```python
from build123d import *

# Parameters (mm, degrees)
F0_W     = 74.9250464141
F0_H     = 66.6232015938
F1_DEPTH = 25.4
F3_DEPTH = 84.074
F4_R     = 1.27


with BuildPart() as f1:
    # F0 (on Top) → F1 (new body)
    with BuildSketch(Plane.XY):
        with Locations((-4.7604274005, 6.0135135427)):
            Rectangle(F0_W, F0_H)
    extrude(amount=F1_DEPTH)

    # F2 (on face) → F3 (cut)
    with BuildSketch(Plane.YZ.offset(32.7020958066)):
        Polygon((25.5974382162, 18.2015541941), (-8.4044123068, 18.2015541941), (1.5848320909, 7.8281089664), (17.7213028073, 7.8281089664), align=None)
    extrude(amount=-F3_DEPTH, mode=Mode.SUBTRACT)

    # F4
    f4_edges = [f1.edges().sort_by_distance(p)[0] for p in [
        (-4.760427, 1.584832, 7.828109),
        (-4.760427, 25.597438, 18.201554),
    ]]
    fillet(f4_edges, radius=F4_R)


solid = f1.part
```
Part model, mm, in its own coordinate system. A direction names the side the tool comes from. Give positions to 0.01 mm unless a question says otherwise; leave off trailing zeros. Write each loop counter-clockwise with the first axis right and the second up, starting at its lowest first coordinate (ties: lowest second). Pieces come first, ordered by that corner, then holes. Notation, with made-up numbers: (77.5, -11) -> (89.5, -11) arc R30 cw to (89.5, 22) -> close; hole circle Ø9 at (73.5, -1). An arc over 180 degrees is marked (long way). Put each result on its own line as item: value. Start each with the question number.
Item 1: Cut at C-C (z = 11). List the corners of the cut face in (x, y), then the cut area to 3 significant figures.
Item 2: Which spindle directions (+Z, -Z, +X, -X, +Y, -Y) get a long thin tool onto all of the face, cutting with end or side? Do faces 1 (the face through (-4.236, -3.664, 13.279)), 2 (the face through (-5, 6, 25.4)). Say none if no direction does.
Item 3: Pin check, flat tip, straight feed: pin 1 Ø25 at (x, y) = (-18.5, 14) entering from -Z. Stop position of the tip, or through.
Item 4: Wall check: L1, parallel to Z at x = -11.5, y = 7; L2, parallel to Z at x = -12, y = 1; L3, parallel to Y at x = -12, z = 9. Give the ranges that are in metal, low to high. Write a range as [from, to].
Item 5: Cut at A-A (y = 7.5). List the corners of the cut face in (x, z).
Item 6: Cut at B-B (x = -17). List the corners of the cut face in (y, z), then the cut area to 3 significant figures.
Item 7: Pull direction Y, two halves, no side cores. Call faces 3 (the face through (-5, 39.325, 13)), 4 (the face through (-5.28, 24.17, 17.51)), 5 (the face through (-5, -27.298, 13)): pulls with the +Y half, pulls with the -Y half, needs draft (parallel to the pull), parting line crosses it, or undercut.
Answer list:
1. outline: (-42.22, -27.3) -> (32.7, -27.3) -> (32.7, -1.47) -> (-42.22, -1.47) -> close; (-42.22, 20.13) -> (32.7, 20.13) -> (32.7, 39.33) -> (-42.22, 39.33) -> close
1. area: 3,370 mm2
2. face 1: +X, -X
2. face 2: +Z, +X, -X, +Y, -Y
3. pin 1: stops at z = 0
4. L1: z = [0, 7.83], [18.2, 25.4]
4. L2: z = [0, 8.44], [18.2, 25.4]
4. L3: y = [-27.3, 0.46], [18.61, 39.33]
5. outline: (-42.22, 0) -> (32.7, 0) -> (32.7, 7.83) -> (-42.22, 7.83) -> close; (-42.22, 18.2) -> (32.7, 18.2) -> (32.7, 25.4) -> (-42.22, 25.4) -> close
6. outline: (-27.3, 0) -> (39.33, 0) -> (39.33, 25.4) -> (-27.3, 25.4) -> close; hole (-8.4, 18.2) -> (1.21, 8.22) arc R1.27 ccw to (2.12, 7.83) -> (17.72, 7.83) -> (24.05, 16.16) arc R1.27 ccw to (23.04, 18.2) -> close
6. area: 1,430 mm2
7. face 3: pulls with the +Y half
7. face 4: undercut
7. face 5: pulls with the -Y half
